```python
from build123d import *

# Parameters (mm, degrees)
BOSS_EXTRUDE1_DEPTH = 20
BOSS_EXTRUDE2_DEPTH = 20
CUT_EXTRUDE1_DEPTH  = 20
SKETCH4_R           = 3.175
CUT_EXTRUDE2_DEPTH  = 4
SKETCH5_W           = 20
SKETCH5_H           = 20
SKETCH5_R           = 3.175
BOSS_EXTRUDE3_DEPTH = 5
BOSS_EXTRUDE4_DEPTH = 20
CUT_EXTRUDE3_START  = -6
CUT_EXTRUDE3_DEPTH  = 2.5
SKETCH9_R           = 1.7
CUT_EXTRUDE4_DEPTH  = 20.237


with BuildPart() as part:
    # Sketch1 → Boss-Extrude1 (new body)
    with BuildSketch(Plane.XY):
        with BuildLine():
            ThreePointArc((-3.138, 8.25), (-2.60201306, 8.47201306), (-2.38, 9.008))
            Line((-2.38, 9.008), (-2.38, 9.492))
            Line((-2.38, 9.492), (-2.38, 13.492))
            Line((-2.38, 13.492), (13.492, 13.492))
            Line((13.492, 13.492), (13.492, -2.38))
            Line((13.492, -2.38), (9.492, -2.38))
            Line((9.492, -2.38), (9.008, -2.38))
            ThreePointArc((9.008, -2.38), (8.47201306, -2.60201306), (8.25, -3.138))
            Line((8.25, -3.138), (8.25, -5.487))
            ThreePointArc((8.25, -5.487), (8.17443355, -5.66943355), (7.992, -5.745))
            Line((7.992, -5.745), (7.266240833, -5.745))
            ThreePointArc((7.266240833, -5.745), (7.167508508, -5.725360919), (7.083807284, -5.66943355))
            Line((7.083807284, -5.66943355), (3.98056645, -2.566192716))
            ThreePointArc((3.98056645, -2.566192716), (3.924639081, -2.482491492), (3.905, -2.383759167))
            Line((3.905, -2.383759167), (3.905, 2.38407951))
            ThreePointArc((3.905, 2.38407951), (3.924639081, 2.482811836), (3.98056645, 2.56651306))
            Line((3.98056645, 2.56651306), (7.08348694, 5.66943355))
            ThreePointArc((7.08348694, 5.66943355), (7.167188164, 5.725360919), (7.26592049, 5.745))
            Line((7.26592049, 5.745), (7.992, 5.745))
            ThreePointArc((7.992, 5.745), (8.17443355, 5.66943355), (8.25, 5.487))
            Line((8.25, 5.487), (8.25, 3.138))
            ThreePointArc((8.25, 3.138), (8.47201306, 2.60201306), (9.008, 2.38))
            Line((9.008, 2.38), (9.492, 2.38))
            ThreePointArc((9.492, 2.38), (10.02798694, 2.60201306), (10.25, 3.138))
            Line((10.25, 3.138), (10.25, 8.5))
            ThreePointArc((10.25, 8.5), (9.737436867, 9.737436867), (8.5, 10.25))
            Line((8.5, 10.25), (3.138, 10.25))
            ThreePointArc((3.138, 10.25), (2.60201306, 10.02798694), (2.38, 9.492))
            Line((2.38, 9.492), (2.38, 9.008))
            ThreePointArc((2.38, 9.008), (2.60201306, 8.47201306), (3.138, 8.25))
            Line((3.138, 8.25), (5.487, 8.25))
            ThreePointArc((5.487, 8.25), (5.66943355, 8.17443355), (5.745, 7.992))
            Line((5.745, 7.992), (5.745, 7.266240833))
            ThreePointArc((5.745, 7.266240833), (5.725360919, 7.167508508), (5.66943355, 7.083807284))
            Line((5.66943355, 7.083807284), (2.566192716, 3.98056645))
            ThreePointArc((2.566192716, 3.98056645), (2.482491492, 3.924639081), (2.383759167, 3.905))
            Line((2.383759167, 3.905), (-2.38407951, 3.905))
            ThreePointArc((-2.38407951, 3.905), (-2.482811836, 3.924639081), (-2.56651306, 3.98056645))
            Line((-2.56651306, 3.98056645), (-5.66943355, 7.08348694))
            ThreePointArc((-5.66943355, 7.08348694), (-5.725360919, 7.167188164), (-5.745, 7.26592049))
            Line((-5.745, 7.26592049), (-5.745, 7.992))
            ThreePointArc((-5.745, 7.992), (-5.66943355, 8.17443355), (-5.487, 8.25))
            Line((-5.487, 8.25), (-3.138, 8.25))
        make_face()
    extrude(amount=-BOSS_EXTRUDE1_DEPTH)

    # Sketch2 → Boss-Extrude2 (add)
    with BuildSketch(Plane.XY):
        Polygon((13.492, 13.492), (237.62, 13.492), (237.62, 9.492), (13.492, -2.38), align=None)
    extrude(amount=-BOSS_EXTRUDE2_DEPTH)

    # Sketch3 → Cut-Extrude1 (cut)
    with BuildSketch(Plane.XY):
        Polygon((237.62, 9.492), (217.62, 9.492), (217.62, 8.432605368), align=None)
    extrude(amount=-CUT_EXTRUDE1_DEPTH, mode=Mode.SUBTRACT)

    # Sketch4 → Cut-Extrude2 (cut)
    with BuildSketch(Plane.XZ.offset(-9.492)):
        with Locations((227.62, -10)):
            Circle(SKETCH4_R)
    extrude(amount=-CUT_EXTRUDE2_DEPTH, mode=Mode.SUBTRACT)

    # Sketch5 → Boss-Extrude3 (add)
    with BuildSketch(Plane.XZ.offset(-9.492)):
        with Locations((227.62, -10)):
            Rectangle(SKETCH5_W, SKETCH5_H)
        with Locations((227.62, -10)):
            Circle(SKETCH5_R, mode=Mode.SUBTRACT)
    extrude(amount=BOSS_EXTRUDE3_DEPTH)

    # Sketch6 → Boss-Extrude4 (add)
    with BuildSketch(Plane.XY):
        Polygon((13.492, -2.38), (217.62, 4.492), (217.62, 8.432605368), align=None)
    extrude(amount=-BOSS_EXTRUDE4_DEPTH)

    # Sketch8 → Cut-Extrude3 (cut)
    with BuildSketch(Plane(origin=(0, 13.492, 0), x_dir=(1, 0, 0), z_dir=(0, 1, 0)).offset(CUT_EXTRUDE3_START)):
        Polygon((2.383759167, 0), (-2.38407951, 0), (-2.800160172, 0), (-2.800160172, 4.383419246), (-2.800160172, 7.616580754), (-0.000160172, 9.233161507), (2.799839828, 7.616580754), (2.799839828, 4.383419246), (2.799839828, 0), align=None)
    extrude(amount=-CUT_EXTRUDE3_DEPTH, mode=Mode.SUBTRACT)

    # Sketch9 → Cut-Extrude4 (cut, through all)
    with BuildSketch(Plane(origin=(0, 13.492, 0), x_dir=(1, 0, 0), z_dir=(0, 1, 0))):
        with Locations((-0.000160172, 6)):
            Circle(SKETCH9_R)
    extrude(amount=-CUT_EXTRUDE4_DEPTH, mode=Mode.SUBTRACT)


solid = part.part
```
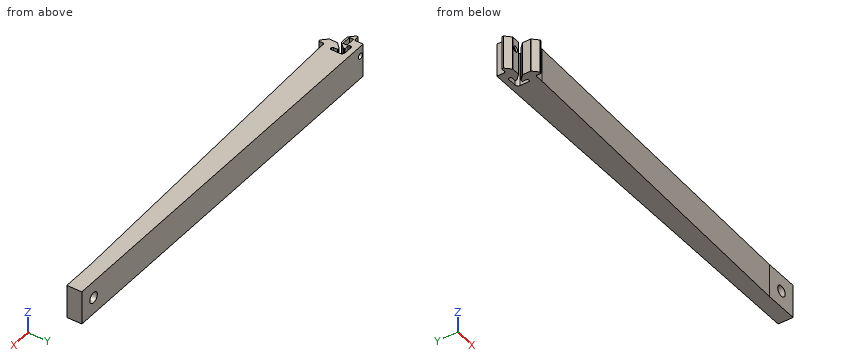
Work out the finished part from the listing and answer in its coordinate system (mm). Give positions to 0.01 mm unless a question says otherwise; leave off trailing zeros. Loops run counter-clockwise (first coordinate to the right, second up) from the corner with the lowest first, then second, coordinate; pieces in that order, holes last. Notation, with made-up numbers: (-9.5, 24.25) -> (31.5, 24.25) arc R26 ccw to (31.5, 43.25) -> close; hole circle Ø4 at (-40, -1). An arc over 180 degrees is marked (long way). Put each result on its own line as item: value. Start each with the question number.
Item 1: The part is cut by section A-A (x = 227.62). Give the vertices of the cut face in (y, z) (3 decimals).
Item 2: Each of these flat-tipped pins is pushed along its axis until it touches: P1, Ø4, axis at x = 0, z = -6, coming from the -Y side (3 decimals); P2, Ø2.5, axis at y = -1, z = -5.5, coming from the -X side (3 decimals); P3, Ø3, axis at y = 6, z = -3.5, coming from the -X side (3 decimals); P4, Ø1, axis at x = 47, y = -2.5, coming from the -Z side. Where does it stop, or does it pass through?
Item 3: The part is cut by section C-C (x = 63). Give the vertices of the cut face in (y, z), then the cut area to 3 significant figures.
Item 4: Find the intervals of material crossed by L1, parallel to X at y = 12.5, z = -6.25; L2, parallel to X at y = 5.5, z = -5.25; L3, parallel to X at y = 8.95, z = -6, in increasing order. Write a range as [from, to].
Item 5: The part is cut by section B-B (x = 151). Give the vertices of the cut face in (y, z), then the cut area to 3 significant figures.
Answers below:
1. outline: (4.492, -20) -> (13.492, -20) -> (13.492, -13.175) -> (4.492, -13.175) -> close; (4.492, -6.825) -> (13.492, -6.825) -> (13.492, 0) -> (4.492, 0) -> close
2. P1: y = 3.905
2. P2: x = 3.905
2. P3: x = -5.745
2. P4: through
3. outline: (-0.71, -20) -> (13.49, -20) -> (13.49, 0) -> (-0.71, 0) -> close
3. area: 284 mm2
4. L1: [-2.38, -1.68], [1.68, 237.62]
4. L2: [-4.09, -2.8], [2.8, 4.09], [6.91, 8.25], [10.25, 237.62]
4. L3: [-2.38, -1.7], [1.7, 2.38], [10.19, 237.62]
5. outline: (2.25, -20) -> (13.49, -20) -> (13.49, 0) -> (2.25, 0) -> close
5. area: 225 mm2
